```python
from build123d import *

# Parameters (mm, degrees)
SKETCH_W        = 150
SKETCH_H        = 110
PAD_DEPTH       = 3
SKETCH001_R     = 1.5
SKETCH001_R_2   = 12
SKETCH001_R_3   = 2
SKETCH001_W     = 58.5
SKETCH001_H     = 40
POCKET_DEPTH    = 3.001
SKETCH002_R     = 1.5
SKETCH002_W     = 38.5
SKETCH002_H     = 8
SKETCH002_W_2   = 14
SKETCH002_H_2   = 13.5
SKETCH002_W_3   = 17
POCKET001_DEPTH = 3.001


with BuildPart() as part:
    # Sketch → Pad (new body)
    with BuildSketch(Plane.XZ):
        with Locations((20, -10)):
            Rectangle(SKETCH_W, SKETCH_H)
    extrude(amount=PAD_DEPTH)

    # Sketch001 (on Face5 of Pad) → Pocket (cut, through all)
    with BuildSketch(Plane(origin=(0, 0, 0), x_dir=(1, 0, 0), z_dir=(0, 1, 0))):
        with Locations((-26.5, 5.07)):
            Circle(SKETCH001_R)
        with Locations((-26.5, -35.07)):
            Circle(SKETCH001_R)
        with Locations((66.5, -35.07)):
            Circle(SKETCH001_R)
        with Locations((66.5, 5.07)):
            Circle(SKETCH001_R)
        with Locations((-16.97, -18.72)):
            Circle(SKETCH001_R_2)
        with Locations((-16.97, -0.68)):
            Circle(SKETCH001_R_3)
        with Locations((34.15, -15)):
            Rectangle(SKETCH001_W, SKETCH001_H)
    extrude(amount=-POCKET_DEPTH, mode=Mode.SUBTRACT)

    # Sketch002 (on Face4 of Pocket) → Pocket001 (cut, through all)
    with BuildSketch(Plane(origin=(0, 0, 0), x_dir=(1, 0, 0), z_dir=(0, 1, 0))):
        with Locations((36.45, 25)):
            Circle(SKETCH002_R)
        with Locations((83.55, 25)):
            Circle(SKETCH002_R)
        with Locations((-38.6, 25)):
            Circle(SKETCH002_R)
        with Locations((-13.5, 25)):
            Circle(SKETCH002_R)
        with Locations((60, 25)):
            Rectangle(SKETCH002_W, SKETCH002_H)
        with Locations((11.5, 25)):
            Rectangle(SKETCH002_W_2, SKETCH002_H_2)
        with Locations((-26.05, 25)):
            Rectangle(SKETCH002_W_3, SKETCH002_H)
    extrude(amount=-POCKET001_DEPTH, mode=Mode.SUBTRACT)


solid = part.part
```
Geometry check sheet. Reference: the model listing, model coordinates, mm. A direction names the side the tool comes from. Round coordinates to 2 decimals unless told otherwise and drop trailing zeros. Order: outer loops, then holes, each group sorted by start corner. A loop starts at its lowest first (then second) coordinate and runs counter-clockwise, first axis right, second up. Notation, with made-up numbers: (36, 6.25) - (69, 6.25) arc R24 cw to (69, 39.25) - close; hole circle Ø9 at (-34, 44.25). An arc over 180 degrees is marked (long way). Use a Markdown table: item, result. Add a question column.
1) Section check C-C (y = -0.7). Count the separate pieces of the cut face and the enclosed holes in it, then the cut area to 3 significant figures.
2) Thickness scan on line 1 along Z through (x, y) = (7.5, -1); line 2 along Z through (x, y) = (66.5, -0.7); line 3 along X through (y, z) = (-1.15, 0.68). Record the ranges inside material, lowest first.
3) Section check A-A (x = -38.6). Record the cut outline in (y, z).
4) Set-up check for faces 1 (the flat face through (60, -1, -29)), 2 (the flat face through (19, -1, 45)): record each of +Z, -Z, +X, -X, +Y, -Y from which the full face is reachable in a straight line by a thin tool's end or side.
5) Section check D-D (x = 36.45). Record the cut outline in (y, z), then the cut area to 3 significant figures.
6) Gauge pin test, flat end, axial feed: P1, Ø4, axis at x = 66.5, z = -5.07, coming from the +Y side. Record the tip position at first contact, or that the pin passes through.
7) Section check B-B (z = 18.72). Record the cut outline in (x, y).
8) Mould release check, pull along X, two halves, no side actions. Record for faces 3 (the flat face through (4.5, -1, -25)), 4 (the flat face through (-55, -1, -11)), 5 (the flat face through (95, -1, -11)), 6 (the flat face through (19, -1, -65)): released by +X, released by -X, zero draft, split by the parting line, or undercut.
Established:
| question | item | result |
|---|---|---|
| 1 | separate pieces | 1 |
| 1 | enclosed holes | 14 |
| 1 | area | 13,000 mm2 |
| 2 | line 1 | -65 to -31.75, -18.25 to -5, 35 to 45 |
| 2 | line 2 | -65 to -29, -21 to -6.57, -3.57 to 33.57, 36.57 to 45 |
| 2 | line 3 | -55 to -18.97, -14.97 to 4.9, 63.4 to 95 |
| 3 | outline | (-3, -65) - (0, -65) - (0, -26.5) - (-3, -26.5) - close; (-3, -23.5) - (0, -23.5) - (0, 45) - (-3, 45) - close |
| 4 | face 1 | +Y, -Y |
| 4 | face 2 | +Z, +X, -X, +Y, -Y |
| 5 | outline | (-3, -65) - (0, -65) - (0, -26.5) - (-3, -26.5) - close; (-3, -23.5) - (0, -23.5) - (0, -5) - (-3, -5) - close; (-3, 35) - (0, 35) - (0, 45) - (-3, 45) - close |
| 5 | area | 201 mm2 |
| 6 | P1 | y = 0 |
| 7 | outline | (-55, -3) - (-28.97, -3) - (-28.97, 0) - (-55, 0) - close; (-4.97, -3) - (4.9, -3) - (4.9, 0) - (-4.97, 0) - close; (63.4, -3) - (95, -3) - (95, 0) - (63.4, 0) - close |
| 8 | face 3 | undercut |
| 8 | face 4 | released by -X |
| 8 | face 5 | released by +X |
| 8 | face 6 | zero draft |
